from build123d import *

# Parameters (mm, degrees)
SKETCH1_W           = 125
SKETCH1_H           = 132.5
SKETCH1_W_2         = 95
SKETCH1_H_2         = 70
BOSS_EXTRUDE1_DEPTH = 3
SKETCH2_R           = 5
CUT_EXTRUDE1_DEPTH  = 10
SKETCH3_W           = 5
SKETCH3_H           = 4
SKETCH3_W_2         = 4
SKETCH3_H_2         = 15
SKETCH3_W_3         = 15
BOSS_EXTRUDE2_DEPTH = 3
SKETCH4_W           = 4
SKETCH4_H           = 10
SKETCH4_H_2         = 11
BOSS_EXTRUDE3_DEPTH = 3


with BuildPart() as part:
    # Sketch1 → Boss-Extrude1 (new body)
    with BuildSketch(Plane.XY):
        with Locations((-62.5, 66.25)):
            Rectangle(SKETCH1_W, SKETCH1_H)
        with Locations((-62.5, 82.5)):
            Rectangle(SKETCH1_W_2, SKETCH1_H_2, mode=Mode.SUBTRACT)
    extrude(amount=BOSS_EXTRUDE1_DEPTH)

    # Sketch2 → Cut-Extrude1 (cut)
    with BuildSketch(Plane.XY.offset(3)):
        with Locations((-62.5, 21.25)):
            Circle(SKETCH2_R)
    extrude(amount=-CUT_EXTRUDE1_DEPTH, mode=Mode.SUBTRACT)

    # Sketch3 → Boss-Extrude2 (add)
    with BuildSketch(Plane.XY.offset(3)):
        with Locations((-62.5, 134.5)):
            Rectangle(SKETCH3_W, SKETCH3_H)
        with Locations((2, 20)):
            Rectangle(SKETCH3_W_2, SKETCH3_H_2)
        with Locations((2, 110)):
            Rectangle(SKETCH3_W_2, SKETCH3_H_2)
        with Locations((2, 80)):
            Rectangle(SKETCH3_W_2, SKETCH3_H_2)
        with Locations((2, 50)):
            Rectangle(SKETCH3_W_2, SKETCH3_H_2)
        with Locations((-102.5, 115.5)):
            Rectangle(SKETCH3_W_3, SKETCH3_H)
        with Locations((-127, 80)):
            Rectangle(SKETCH3_W_2, SKETCH3_H_2)
        with Locations((-127, 110)):
            Rectangle(SKETCH3_W_2, SKETCH3_H_2)
        with Locations((-127, 50)):
            Rectangle(SKETCH3_W_2, SKETCH3_H_2)
        with Locations((-127, 20)):
            Rectangle(SKETCH3_W_2, SKETCH3_H_2)
        with Locations((-117.5, 134.5)):
            Rectangle(SKETCH3_W_3, SKETCH3_H)
        with Locations((-7.5, 134.5)):
            Rectangle(SKETCH3_W_3, SKETCH3_H)
        with Locations((-37.5, 134.5)):
            Rectangle(SKETCH3_W_3, SKETCH3_H)
        with Locations((-87.5, 134.5)):
            Rectangle(SKETCH3_W_3, SKETCH3_H)
        with Locations((-22.5, 115.5)):
            Rectangle(SKETCH3_W_3, SKETCH3_H)
        with Locations((-72.5, 115.5)):
            Rectangle(SKETCH3_W_3, SKETCH3_H)
        with Locations((-52.5, 115.5)):
            Rectangle(SKETCH3_W_3, SKETCH3_H)
        with Locations((-52.5, 49.5)):
            Rectangle(SKETCH3_W_3, SKETCH3_H)
        with Locations((-22.5, 49.5)):
            Rectangle(SKETCH3_W_3, SKETCH3_H)
        with Locations((-72.5, 49.5)):
            Rectangle(SKETCH3_W_3, SKETCH3_H)
        with Locations((-102.5, 49.5)):
            Rectangle(SKETCH3_W_3, SKETCH3_H)
    extrude(amount=-BOSS_EXTRUDE2_DEPTH)

    # Sketch4 → Boss-Extrude3 (add)
    with BuildSketch(Plane.XY.offset(3)):
        with Locations((-108, 82.5)):
            Rectangle(SKETCH4_W, SKETCH4_H)
        with Locations((-108, 108)):
            Rectangle(SKETCH4_W, SKETCH4_H_2)
        with Locations((-108, 57)):
            Rectangle(SKETCH4_W, SKETCH4_H_2)
        with Locations((-17, 57)):
            Rectangle(SKETCH4_W, SKETCH4_H_2)
        with Locations((-17, 82.5)):
            Rectangle(SKETCH4_W, SKETCH4_H)
        with Locations((-17, 108)):
            Rectangle(SKETCH4_W, SKETCH4_H_2)
    extrude(amount=-BOSS_EXTRUDE3_DEPTH)


solid = part.part
The listing builds one solid part. Answer for the finished solid, in the listing's coordinates (mm). A direction names the side the tool comes from. Coordinates: 2 decimals unless noted, no trailing zeros. Loops run counter-clockwise (first coordinate to the right, second up) from the corner with the lowest first, then second, coordinate; pieces in that order, holes last.
1) A tool of negligible diameter and unlimited length cuts with its end or side. For faces 1 (the face through (-127, 72.5, 2)), 2 (the face through (-73, 51.5, 2)), 3 (the face through (-65, 134, 2)), from which of +Z, -Z, +X, -X, +Y, -Y can it reach the whole face along a straight path? Write none if from no direction.
2) Find section C-C on x = -98. Write down the section's boundary in (y, z).
3) Find section D-D on z = 1.5. Give the number of separate pieces and of enclosed holes in the cut face, then the cut area to 3 significant figures.
4) Find the intervals of material crossed by L1, parallel to Y at x = -62.5, z = 2.05; L2, parallel to X at y = 89, z = 0.8; L3, parallel to Y at x = -101, z = 2.55, in increasing order.
5) Find section A-A on y = 21.25. Write down the section's boundary in (x, z), then the cut area to 3 significant figures.
6) Flat-ended cylindrical pins translate along their axes: pin 1 Ø1.5 at (y, z) = (134.5, 1.5) entering from -X; pin 2 Ø1.5 at (y, z) = (134, 1) entering from +X; pin 3 Ø8 at (x, y) = (-52, 41.5) entering from -Z. Find the tip coordinate at first contact, or state that the pin passes through.
7) Determine the mould class of faces 4 (the face through (-125, 65, 1)), 5 (the face through (-127, 27.5, 2)), 6 (the face through (-38, 117.5, 1)) for opening direction X: pulls with the +X half, pulls with the -X half, needs draft (parallel to the pull), parting line crosses it, or undercut.
8) Find section B-B on x = -62.5. Write down the section's boundary in (y, z), then the cut area to 4 significant figures.
Values:
1. face 1: +Z, -Z, -X
1. face 2: +Z, -Z
1. face 3: +Z, -Z, +Y
2. outline: (0, 0) - (51.5, 0) - (51.5, 3) - (0, 3) - close; (113.5, 0) - (132.5, 0) - (132.5, 3) - (113.5, 3) - close
3. separate pieces: 1
3. enclosed holes: 2
3. area: 11,300 mm2
4. L1: y = 0 to 16.25, 26.25 to 47.5, 117.5 to 136.5
4. L2: x = -125 to -110, -15 to 0
4. L3: y = 0 to 51.5, 113.5 to 132.5
5. outline: (-129, 0) - (-67.5, 0) - (-67.5, 3) - (-129, 3) - close; (-57.5, 0) - (4, 0) - (4, 3) - (-57.5, 3) - close
5. area: 369 mm2
6. pin 1: stops at x = -125
6. pin 2: stops at x = 0
6. pin 3: stops at z = 0
7. face 4: pulls with the -X half
7. face 5: needs draft
7. face 6: undercut
8. outline: (0, 0) - (16.25, 0) - (16.25, 3) - (0, 3) - close; (26.25, 0) - (47.5, 0) - (47.5, 3) - (26.25, 3) - close; (117.5, 0) - (136.5, 0) - (136.5, 3) - (117.5, 3) - close
8. area: 169.5 mm2
